from build123d import *

# Parameters (mm, degrees)
BOSS_EXTRUDE1_DEPTH = 12
SKETCH3_R           = 1.505
CUT_EXTRUDE2_DEPTH  = 4
SKETCH5_R           = 1.6
CUT_EXTRUDE3_DEPTH  = 4
SKETCH6_W           = 8.02
SKETCH6_H           = 8.02
CUT_EXTRUDE4_DEPTH  = 2
FILLET1_R           = 2
FILLET2_R           = 2
FILLET3_R           = 2
FILLET4_R           = 2
FILLET5_R           = 2
FILLET6_R           = 2


with BuildPart() as part:
    # Sketch1 → Boss-Extrude1 (new body)
    with BuildSketch(Plane(origin=(0, 0, 0), x_dir=(1, 0, 0), z_dir=(0, 1, 0))):
        Polygon((0, 0), (-32, 0), (-32, 50.8), (0, 50.8), (0, 48.8), (-30, 48.8), (-30, 2), (0, 2), align=None)
    extrude(amount=BOSS_EXTRUDE1_DEPTH)

    # Sketch3 → Cut-Extrude2 (cut)
    with BuildSketch(Plane(origin=(0, 0, -50.8), x_dir=(-1, 0, 0), z_dir=(0, 0, -1))):
        with Locations((6.01, 6)):
            Circle(SKETCH3_R)
    extrude(amount=-CUT_EXTRUDE2_DEPTH, mode=Mode.SUBTRACT)

    # Sketch5 → Cut-Extrude3 (cut)
    with BuildSketch(Plane.ZY.offset(32)):
        with Locations((-43.9, 6)):
            Circle(SKETCH5_R)
        with Locations((-6.9, 6)):
            Circle(SKETCH5_R)
    extrude(amount=-CUT_EXTRUDE3_DEPTH, mode=Mode.SUBTRACT)

    # Sketch6 → Cut-Extrude4 (cut)
    with BuildSketch(Plane.XY):
        with Locations((-6.01, 6)):
            Rectangle(SKETCH6_W, SKETCH6_H)
    extrude(amount=-CUT_EXTRUDE4_DEPTH, mode=Mode.SUBTRACT)

    # Fillet1
    fillet1_edges = [part.edges().sort_by_distance(p)[0] for p in [
        (0, 12, -1),
    ]]
    fillet(fillet1_edges, radius=FILLET1_R)

    # Fillet2
    fillet2_edges = [part.edges().sort_by_distance(p)[0] for p in [
        (0, 12, -49.8),
    ]]
    fillet(fillet2_edges, radius=FILLET2_R)

    # Fillet3
    fillet3_edges = [part.edges().sort_by_distance(p)[0] for p in [
        (-30, 6, -2),
    ]]
    fillet(fillet3_edges, radius=FILLET3_R)

    # Fillet4
    fillet4_edges = [part.edges().sort_by_distance(p)[0] for p in [
        (-32, 6, 0),
    ]]
    fillet(fillet4_edges, radius=FILLET4_R)

    # Fillet5
    fillet5_edges = [part.edges().sort_by_distance(p)[0] for p in [
        (-30, 6, -48.8),
    ]]
    fillet(fillet5_edges, radius=FILLET5_R)

    # Fillet6
    fillet6_edges = [part.edges().sort_by_distance(p)[0] for p in [
        (-32, 6, -50.8),
    ]]
    fillet(fillet6_edges, radius=FILLET6_R)


solid = part.part
Geometry check sheet. Reference: the model listing, model coordinates, mm. A direction names the side the tool comes from. Give positions to 0.01 mm unless a question says otherwise; leave off trailing zeros. Loops run counter-clockwise (first coordinate to the right, second up) from the corner with the lowest first, then second, coordinate; pieces in that order, holes last. Notation, with made-up numbers: (78, 43.5) -> (95, 43.5) arc R13 cw to (95, 59.5) -> close; hole circle Ø2 at (-12.75, 46.5). An arc over 180 degrees is marked (long way). Answer in a Markdown table with one row per item. Add a question column.
1) Draft check along Z on faces 1 (the face through (-15, 6, 0)), 2 (the face through (-31, 0, -26)), 3 (the face through (-29.43, 6.08, -2.6)), 4 (the face through (-14, 6, -48.8)). Enter one of: pulls with the +Z half, pulls with the -Z half, needs draft (parallel to the pull), parting line crosses it, or undercut.
2) Cross-section at C-C on y = 6. Record the boundary of the cut face in (x, z) (3 decimals), and give its area (3 significant figures).
3) Material ranges on probe 1 along Y at (x, z) = (-31.3, -6.9); probe 2 along Z at (x, y) = (-22, 1.75); probe 3 along Y at (x, z) = (-6.01, -50.2) (3 decimals), recorded low to high. Write a range as from..to.
4) Set-up check for faces 5 (the face through (-30, 6, -26)), 6 (the face through (-10.02, 6, -1)), 7 (the face through (-0.57, 11.4, -0.99)): record each of +Z, -Z, +X, -X, +Y, -Y from which the full face is reachable in a straight line by a thin tool's end or side.
5) Cross-section at D-D on x = -6.01. Record the boundary of the cut face in (y, z) (3 decimals), and give its area (3 significant figures).
6) Cross-section at A-A on z = -43.9. Record the boundary of the cut face in (x, y), and give its area (3 significant figures).
7) Cross-section at B-B on x = -12. Record the boundary of the cut face in (y, z).
8) Gauge pin test, flat ends, axial feed: P1, Ø0.6, axis at y = 4.5, z = -1.5, coming from the -X side; P2, Ø1.5, axis at y = 3.5, z = -32, coming from the +X side; P3, Ø1, axis at x = -5.5, z = -1.5, coming from the -Y side. Record the tip position at first contact, or that the pin passes through.
Outcome:
| question | item | result |
|---|---|---|
| 1 | face 1 | pulls with the +Z half |
| 1 | face 2 | needs draft |
| 1 | face 3 | undercut |
| 1 | face 4 | undercut |
| 2 | outline | (-32, -48.8) arc R2 ccw to (-30, -50.8) -> (-7.515, -50.8) -> (-7.515, -48.8) -> (-28, -48.8) arc R2 cw to (-30, -46.8) -> (-30, -45.5) -> (-32, -45.5) -> close; (-32, -42.3) -> (-30, -42.3) -> (-30, -8.5) -> (-32, -8.5) -> close; (-32, -5.3) -> (-30, -5.3) -> (-30, -4) arc R2 cw to (-28, -2) -> (-10.02, -2) -> (-10.02, 0) -> (-30, 0) arc R2 ccw to (-32, -2) -> close; (-4.505, -50.8) -> (0, -50.8) -> (0, -48.8) -> (-4.505, -48.8) -> close; (-2, -2) -> (0, -2) -> (0, 0) -> (-2, 0) -> close |
| 2 | area | 187 mm^2 |
| 3 | probe 1 | y = 0..4.4, 7.6..12 |
| 3 | probe 2 | z = -50.8..-48.8, -2..0 |
| 3 | probe 3 | y = 0..4.495, 7.505..12 |
| 4 | face 5 | +X, +Y, -Y |
| 4 | face 6 | +Z |
| 4 | face 7 | +Z, -Z, +X, +Y |
| 5 | outline | (0, -50.8) -> (4.495, -50.8) -> (4.495, -48.8) -> (0, -48.8) -> close; (0, -2) -> (1.99, -2) -> (1.99, 0) -> (0, 0) -> close; (7.505, -50.8) -> (12, -50.8) -> (12, -48.8) -> (7.505, -48.8) -> close; (10.01, -2) -> (12, -2) -> (12, 0) -> (10.01, 0) -> close |
| 5 | area | 25.9 mm^2 |
| 6 | outline | (-32, 0) -> (-30, 0) -> (-30, 4.4) -> (-32, 4.4) -> close; (-32, 7.6) -> (-30, 7.6) -> (-30, 12) -> (-32, 12) -> close |
| 6 | area | 17.6 mm^2 |
| 7 | outline | (0, -50.8) -> (12, -50.8) -> (12, -48.8) -> (0, -48.8) -> close; (0, -2) -> (12, -2) -> (12, 0) -> (0, 0) -> close |
| 8 | P1 | stops at x = -31.99 |
| 8 | P2 | stops at x = -30 |
| 8 | P3 | stops at y = 0 |
